Read the model definition and answer for the solid it produces. Units are mm, in the model's axes. A direction names the side the tool comes from. Give positions to 0.01 mm unless a question says otherwise; leave off trailing zeros. Order: outer loops, then holes, each group sorted by start corner. A loop starts at its lowest first (then second) coordinate and runs counter-clockwise, first axis right, second up. Notation, with made-up numbers: M 10,20.25 L 21,20.25 A9 ccw 21,37.25 Z; hole C 2,40.5 d5. An arc over 180 degrees is marked long. One line per item, written item: value. Start each with the question number.
from build123d import *

# Parameters (mm, degrees)
SKETCH1_R           = 3
BOSS_EXTRUDE1_DEPTH = 9


with BuildPart() as part:
    # Sketch1 → Boss-Extrude1 (new, symmetric)
    with BuildSketch(Plane.XY):
        with BuildLine():
            Line((6, 0), (6, -87))
            ThreePointArc((6, -87), (0, -93), (-6, -87))
            Line((-6, -87), (-6, 0))
            ThreePointArc((-6, 0), (0, 6), (6, 0))
        make_face()
        with Locations((0, -87)):
            Circle(SKETCH1_R, mode=Mode.SUBTRACT)
        Circle(SKETCH1_R, mode=Mode.SUBTRACT)
        with Locations((0, -43.5)):
            Circle(SKETCH1_R, mode=Mode.SUBTRACT)
        with BuildLine():
            Line((3, -10), (3, -33.5))
            ThreePointArc((3, -33.5), (0, -36.5), (-3, -33.5))
            Line((-3, -33.5), (-3, -10))
            ThreePointArc((-3, -10), (0, -7), (3, -10))
        make_face(mode=Mode.SUBTRACT)
        with BuildLine():
            Line((3, -53.5), (3, -77))
            ThreePointArc((3, -77), (0, -80), (-3, -77))
            Line((-3, -77), (-3, -53.5))
            ThreePointArc((-3, -53.5), (0, -50.5), (3, -53.5))
        make_face(mode=Mode.SUBTRACT)
    extrude(amount=BOSS_EXTRUDE1_DEPTH, both=True)


solid = part.part
Q1. A tool of negligible diameter and unlimited length cuts with its end or side. For faces 5 (the flat face through (3, -22, 0)), 6 (the cylindrical face through (0, 6, 0)), from which of +Z, -Z, +X, -X, +Y, -Y can it reach the whole face along a straight path? Write none if from no direction.
Q2. Determine the mould class of faces 1 (the cylindrical face through (-0.391, -40.526, -0.126)), 2 (the flat face through (6, -43, 0)), 3 (the flat face through (-6, -44, 0)), 4 (the flat face through (4, -43, -9)) for opening direction X: released by +X, released by -X, zero draft, split by the parting line, or undercut.
Q3. Find section B-B, the plane y = -43.5. Give the vertices of the cut face in (x, z).
Q4. Find section A-A, the plane z = -3.25. Give the vertices of the cut face in (x, y), then the cut area to 3 significant figures.
Q5. Each of these flat-tipped pins is pushed along its axis until it touches: pin 1 (5.5 mm diameter, centred on x = 0, y = -87, fed in from +Z); pin 2 (5 mm diameter, centred on x = 1.5, y = -32, fed in from +Z); pin 3 (6 mm diameter, centred on x = 5, z = -1, fed in from +Y); pin 4 (1.5 mm diameter, centred on x = -4.5, z = 6, fed in from -Y). Where does it stop, or does it pass through?
Q6. Consider probe 1 along Y at (x, z) = (0, -0.5); probe 2 along X at (y, z) = (-14, 3); probe 3 along Y at (x, z) = (1, -4.75). Determine where each line is inside the solid, lowest interval first.
Evaluation:
1. face 5: +Z, -Z
1. face 6: +Z, -Z, +Y
2. face 1: undercut
2. face 2: released by +X
2. face 3: released by -X
2. face 4: zero draft
3. outline: M -6,-9 L -3,-9 L -3,9 L -6,9 Z; M 3,-9 L 6,-9 L 6,9 L 3,9 Z
4. outline: M -6,-87 A6 ccw 6,-87 L 6,0 A6 ccw -6,0 Z; hole C 0,-87 d6; hole M -3,-77 A3 ccw 3,-77 L 3,-53.5 A3 ccw -3,-53.5 Z; hole C 0,-43.5 d6; hole M -3,-33.5 A3 ccw 3,-33.5 L 3,-10 A3 ccw -3,-10 Z; hole C 0,0 d6
4. area: 734 mm2
5. pin 1: through
5. pin 2: z = 9
5. pin 3: y = 5.66
5. pin 4: y = -91.68
6. probe 1: -93 to -90, -84 to -80, -50.5 to -46.5, -40.5 to -36.5, -7 to -3, 3 to 6
6. probe 2: -6 to -3, 3 to 6
6. probe 3: -92.92 to -89.83, -84.17 to -79.83, -50.67 to -46.33, -40.67 to -36.33, -7.17 to -2.83, 2.83 to 5.92
